```python
from build123d import *

# Parameters (mm, degrees)
CASING_R            = 8
CASING_R_2          = 4
BOSS_EXTRUDE1_DEPTH = 10
CUT_EXTRUDE1_REACH  = 17.1
NOTCH_W             = 1.5
NOTCH_H             = 2.2


with BuildPart() as part:
    # Casing → Boss-Extrude1 (new body)
    with BuildSketch(Plane(origin=(0, 0, 0), x_dir=(1, 0, 0), z_dir=(0, 1, 0))):
        with Locations(Location((0, 0, 0), (0, 0, 270))):
            Circle(CASING_R)
        with Locations(Location((0, 0, 0), (0, 0, 270))):
            Circle(CASING_R_2, mode=Mode.SUBTRACT)
    extrude(amount=BOSS_EXTRUDE1_DEPTH)

    # Notch → Cut-Extrude1 (cut, up to next)
    with BuildSketch(Plane(origin=(0, 0, 0), x_dir=(1, 0, 0), z_dir=(0, 1, 0)), mode=Mode.PRIVATE) as cut_extrude1_sk1:
        with Locations((0, 5.029058411)):
            Rectangle(NOTCH_W, NOTCH_H)
    cut_extrude1_tool1 = extrude(cut_extrude1_sk1.sketch, amount=CUT_EXTRUDE1_REACH, mode=Mode.PRIVATE) & part.part
    # Notch → Cut-Extrude1 (cut, up to next)
    with BuildSketch(Plane(origin=(0, 0, 0), x_dir=(1, 0, 0), z_dir=(0, 1, 0)), mode=Mode.PRIVATE) as cut_extrude1_sk2:
        Polygon((-2.604244211, 3.036101462), (-4.324273473, 4.407779026), (-5.259508175, 3.235031803), (-3.539478914, 1.863354239), align=None)
    cut_extrude1_tool2 = extrude(cut_extrude1_sk2.sketch, amount=CUT_EXTRUDE1_REACH, mode=Mode.PRIVATE) & part.part
    # Notch → Cut-Extrude1 (cut, up to next)
    with BuildSketch(Plane(origin=(0, 0, 0), x_dir=(1, 0, 0), z_dir=(0, 1, 0)), mode=Mode.PRIVATE) as cut_extrude1_sk3:
        Polygon((-3.997439414, -0.143101813), (-6.142280821, -0.632647868), (-5.80849942, -2.095039736), (-3.663658013, -1.605493681), align=None)
    cut_extrude1_tool3 = extrude(cut_extrude1_sk3.sketch, amount=CUT_EXTRUDE1_REACH, mode=Mode.PRIVATE) & part.part
    # Notch → Cut-Extrude1 (cut, up to next)
    with BuildSketch(Plane(origin=(0, 0, 0), x_dir=(1, 0, 0), z_dir=(0, 1, 0)), mode=Mode.PRIVATE) as cut_extrude1_sk4:
        Polygon((-2.380481206, -3.214546504), (-3.335025432, -5.196678014), (-1.98357213, -5.847503623), (-1.029027904, -3.865372113), align=None)
    cut_extrude1_tool4 = extrude(cut_extrude1_sk4.sketch, amount=CUT_EXTRUDE1_REACH, mode=Mode.PRIVATE) & part.part
    # Notch → Cut-Extrude1 (cut, up to next)
    with BuildSketch(Plane(origin=(0, 0, 0), x_dir=(1, 0, 0), z_dir=(0, 1, 0)), mode=Mode.PRIVATE) as cut_extrude1_sk5:
        Polygon((1.029027904, -3.865372113), (1.98357213, -5.847503623), (3.335025432, -5.196678014), (2.380481206, -3.214546504), align=None)
    cut_extrude1_tool5 = extrude(cut_extrude1_sk5.sketch, amount=CUT_EXTRUDE1_REACH, mode=Mode.PRIVATE) & part.part
    # Notch → Cut-Extrude1 (cut, up to next)
    with BuildSketch(Plane(origin=(0, 0, 0), x_dir=(1, 0, 0), z_dir=(0, 1, 0)), mode=Mode.PRIVATE) as cut_extrude1_sk6:
        Polygon((3.663658013, -1.605493681), (5.80849942, -2.095039736), (6.142280821, -0.632647868), (3.997439414, -0.143101813), align=None)
    cut_extrude1_tool6 = extrude(cut_extrude1_sk6.sketch, amount=CUT_EXTRUDE1_REACH, mode=Mode.PRIVATE) & part.part
    # Notch → Cut-Extrude1 (cut, up to next)
    with BuildSketch(Plane(origin=(0, 0, 0), x_dir=(1, 0, 0), z_dir=(0, 1, 0)), mode=Mode.PRIVATE) as cut_extrude1_sk7:
        Polygon((3.539478914, 1.863354239), (5.259508175, 3.235031803), (4.324273473, 4.407779026), (2.604244211, 3.036101462), align=None)
    cut_extrude1_tool7 = extrude(cut_extrude1_sk7.sketch, amount=CUT_EXTRUDE1_REACH, mode=Mode.PRIVATE) & part.part
    add(cut_extrude1_tool1.solids().sort_by_distance((0, 0, -5.029058))[0], mode=Mode.SUBTRACT)
    add(cut_extrude1_tool2.solids().sort_by_distance((-3.931876, 0, -3.135567))[0], mode=Mode.SUBTRACT)
    add(cut_extrude1_tool3.solids().sort_by_distance((-4.902969, 0, 1.119071))[0], mode=Mode.SUBTRACT)
    add(cut_extrude1_tool4.solids().sort_by_distance((-2.182027, 0, 4.531025))[0], mode=Mode.SUBTRACT)
    add(cut_extrude1_tool5.solids().sort_by_distance((2.182027, 0, 4.531025))[0], mode=Mode.SUBTRACT)
    add(cut_extrude1_tool6.solids().sort_by_distance((4.902969, 0, 1.119071))[0], mode=Mode.SUBTRACT)
    add(cut_extrude1_tool7.solids().sort_by_distance((3.931876, 0, -3.135567))[0], mode=Mode.SUBTRACT)


solid = part.part
```
CAD build for the part. Positions are in the model's coordinates, mm. A direction names the side the tool comes from. Round coordinates to 2 decimals unless told otherwise and drop trailing zeros. Order: outer loops, then holes, each group sorted by start corner. A loop starts at its lowest first (then second) coordinate and runs counter-clockwise, first axis right, second up. Notation, with made-up numbers: (-12.75, 54.5) -> (18.25, 54.5) arc R19 ccw to (18.25, 72.5) -> close; hole circle Ø6 at (32.5, 31.25). An arc over 180 degrees is marked (long way). One line per question, with ' | ' between items.
Q1. Two-plate mould, pull along X, no slides. Class faces 3 (the cylindrical face through (0, 5, 4)), 4 (the cylindrical face through (-7.81, 4.93, -1.73)), 5 (the flat face through (4, 0, 2)): released by +X, released by -X, zero draft, split by the parting line, or undercut.
Completed:
face 3: undercut | face 4: split by the parting line | face 5: zero draft
Q2. Which spindle directions (+Z, -Z, +X, -X, +Y, -Y) get a long thin tool onto all of the face, cutting with end or side? Do faces 1 (the flat face through (-5.055, 4.93, 0.384)), 2 (the flat face through (4, 10, 2)). Say none if no direction does.
Completed:
face 1: +Y, -Y | face 2: +Z, -Z, +X, -X, +Y
Q3. Slice it at A-A (x = 0). Write the cut outline in (y, z).
Completed:
outline: (0, -8) -> (10, -8) -> (10, -6.13) -> (0, -6.13) -> close; (0, 4) -> (10, 4) -> (10, 8) -> (0, 8) -> close
Q4. Drop flat-ended pins along their axis: pin 1 (2 mm diameter, centred on y = 7.5, z = 0.5, fed in from -X); pin 2 (1.1 mm diameter, centred on y = 5, z = -4.5, fed in from +X); pin 3 (2 mm diameter, centred on x = -4.5, y = 5, fed in from +Z); pin 4 (2.5 mm diameter, centred on y = 4.5, z = -5.5, fed in from -X). Give the stop position or say it passes through.
Completed:
pin 1: stops at x = -8 | pin 2: stops at x = 6.96 | pin 3: stops at z = 7.19 | pin 4: stops at x = -6.78
Q5. Slice it at C-C (z = -5.5). Write the cut outline in (x, y).
Completed:
outline: (-5.81, 0) -> (-0.75, 0) -> (-0.75, 10) -> (-5.81, 10) -> close; (0.75, 0) -> (5.81, 0) -> (5.81, 10) -> (0.75, 10) -> close
Q6. Probe probe 1 along Z at (x, y) = (2.75, 9.25); probe 2 along X at (y, z) = (1.5, -4.25); probe 3 along X at (y, z) = (2.5, 5.5). List the from-to ranges inside material, lowest first.
Completed:
probe 1: z = -7.51 to -3.15, 2.9 to 3.98, 5.48 to 7.51 | probe 2: x = -6.78 to -4.45, -4.13 to -0.75, 0.75 to 4.13, 4.45 to 6.78 | probe 3: x = -5.81 to -2.71, -1.82 to 1.82, 2.71 to 5.81
